```python
from build123d import *

# Parameters (mm, degrees)
SKETCH1_R           = 6
BOSS_EXTRUDE1_DEPTH = 20
SKETCH3_R           = 2.9
CUT_EXTRUDE1_DEPTH  = 26
BOSS_EXTRUDE2_DEPTH = 2
BOSS_EXTRUDE3_DEPTH = 2
SKETCH6_W           = 1
SKETCH6_H           = 20
CUT_EXTRUDE2_DEPTH  = 17
SKETCH7_R           = 2.9
CUT_EXTRUDE3_DEPTH  = 17


with BuildPart() as part:
    # Sketch1 → Boss-Extrude1 (new body)
    with BuildSketch(Plane(origin=(0, 0, 0), x_dir=(1, 0, 0), z_dir=(0, 1, 0))):
        with Locations(Location((0, 0, 0), (0, 0, 270))):
            Circle(SKETCH1_R)
    extrude(amount=BOSS_EXTRUDE1_DEPTH)

    # Sketch3 → Cut-Extrude1 (cut)
    with BuildSketch(Plane(origin=(0, 20, 0), x_dir=(1, 0, 0), z_dir=(0, 1, 0))):
        with Locations(Location((0, 0, 0), (0, 0, 270))):
            Circle(SKETCH3_R)
    extrude(amount=-CUT_EXTRUDE1_DEPTH, mode=Mode.SUBTRACT)

    # Sketch4 → Boss-Extrude2 (add)
    with BuildSketch(Plane(origin=(-2.5, 0, 0), x_dir=(0, 0, -1), z_dir=(1, 0, 0))):
        Polygon((6, 20), (16, 20), (16, 0), (6, 0), (4.545153511, 0), (4.545153511, 20), align=None)
    extrude(amount=BOSS_EXTRUDE2_DEPTH)

    # Sketch5 → Boss-Extrude3 (add)
    with BuildSketch(Plane(origin=(2.5, 0, 0), x_dir=(0, 0, -1), z_dir=(1, 0, 0))):
        Polygon((6, 20), (16, 20), (16, 0), (6, 0), (4.211348031, 0), (4.211348031, 20), align=None)
    extrude(amount=-BOSS_EXTRUDE3_DEPTH)

    # Sketch6 → Cut-Extrude2 (cut)
    with BuildSketch(Plane(origin=(0, 0, -16), x_dir=(-1, 0, 0), z_dir=(0, 0, -1))):
        with Locations((0, 10)):
            Rectangle(SKETCH6_W, SKETCH6_H)
    extrude(amount=-CUT_EXTRUDE2_DEPTH, mode=Mode.SUBTRACT)

    # Sketch7 → Cut-Extrude3 (cut)
    with BuildSketch(Plane.ZY.offset(2.5)):
        with Locations((-10.727178029, 10)):
            Circle(SKETCH7_R)
    extrude(amount=-CUT_EXTRUDE3_DEPTH, mode=Mode.SUBTRACT)


solid = part.part
```
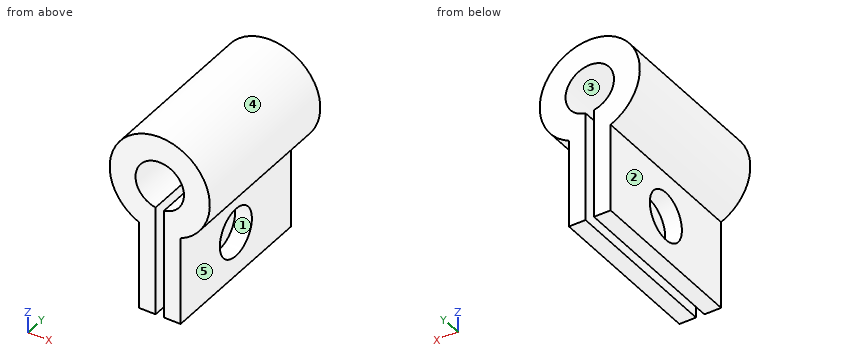
Geometry: final body of the model. Coordinates: model frame, mm. Face numbers are marked on the shaded views. A direction names the side the tool comes from. Coordinates: 2 decimals unless noted, no trailing zeros. Order: outer loops, then holes, each group sorted by start corner. A loop starts at its lowest first (then second) coordinate and runs counter-clockwise, first axis right, second up. Notation, with made-up numbers: (-33, 45.5) - (22, 45.5) arc R15 ccw to (22, 50.5) - close; hole circle Ø7 at (3.25, 6). An arc over 180 degrees is marked (long way). Write each question's results on one line, items separated by ' | '.
1) Pin query (flat end, axial travel): pin 1 (5 mm diameter, centred on x = 3, z = -9.5, fed in from +Y); pin 2 (10.5 mm diameter, centred on y = 12.5, z = -9, fed in from -X); pin 3 (6.5 mm diameter, centred on y = 9.5, z = -9.5, fed in from +X); pin 4 (10 mm diameter, centred on y = 4, z = -12, fed in from -X). Return the tip coordinate at first contact, or that it passes through.
Results list:
pin 1: y = 20 | pin 2: x = -4.68 | pin 3: x = 2.5 | pin 4: x = -2.5
2) Section A-A, the plane y = 10. Return loops of the section in (x, z).
Results list:
outline: (-2.5, -16) - (-0.5, -16) - (-0.5, -13.63) - (-2.5, -13.63) - close; (-2.5, -7.83) - (-0.5, -7.83) - (-0.5, -2.86) arc R2.9 cw (long way) to (0.5, -2.86) - (0.5, -7.83) - (2.5, -7.83) - (2.5, -5.45) arc R6 ccw (long way) to (-2.5, -5.45) - close; (0.5, -16) - (2.5, -16) - (2.5, -13.63) - (0.5, -13.63) - close
3) Section C-C, the plane x = 1.5. Return loops of the section in (y, z).
Results list:
outline: (0, -16) - (20, -16) - (20, -2.48) - (0, -2.48) - close; (0, 2.48) - (20, 2.48) - (20, 5.81) - (0, 5.81) - close; hole circle Ø5.8 at (10, -10.73)
4) Pull-direction query (Z, two-part tool) for the marked faces 3, 4 and 5; classes: pulls with the +Z half, pulls with the -Z half, needs draft (parallel to the pull), parting line crosses it, or undercut.
Results list:
face 3: undercut | face 4: parting line crosses it | face 5: needs draft
5) Section B-B, the plane z = 0. Return loops of the section in (x, y).
Results list:
outline: (-6, 0) - (-2.9, 0) - (-2.9, 20) - (-6, 20) - close; (2.9, 0) - (6, 0) - (6, 20) - (2.9, 20) - close
6) Line query: line 1 (X direction, y = 9, z = 0); line 2 (Z direction, x = -1.75, y = 12); line 3 (Z direction, x = 2, y = 8.75). Output: solid intervals per line, ascending. Write a range as from..to.
Results list:
line 1: -6..-2.9, 2.9..6 | line 2: -16..-12.83, -8.63..-2.31, 2.31..5.74 | line 3: -16..-13.34, -8.11..-2.1, 2.1..5.66
7) Section D-D, the plane z = -9.5. Return loops of the section in (x, y), plus the area to 3 significant figures.
Results list:
outline: (-2.5, 0) - (-0.5, 0) - (-0.5, 7.37) - (-2.5, 7.37) - close; (-2.5, 12.63) - (-0.5, 12.63) - (-0.5, 20) - (-2.5, 20) - close; (0.5, 0) - (2.5, 0) - (2.5, 7.37) - (0.5, 7.37) - close; (0.5, 12.63) - (2.5, 12.63) - (2.5, 20) - (0.5, 20) - close | area: 59.0 mm^2
8) Set-up query: the marked faces 1 and 2. Return all of +Z, -Z, +X, -X, +Y, -Y with unobstructed straight access to the full face (end or side cutting, diameter ignored); none if empty.
Results list:
face 1: +X, -X | face 2: -Z, -X, +Y, -Y
